Print and shaded views of the part. All mm, measured from the part's lowest x, y and z. Give positions to 0.01 mm unless a question says otherwise; leave off trailing zeros. Order: outer loops, then holes, each group sorted by start corner. A loop starts at its lowest first (then second) coordinate and runs counter-clockwise, first axis right, second up. Notation, with made-up numbers: (42.25, -22) - (85.25, -22) arc R31 cw to (85.25, 13) - close; hole circle Ø7 at (20.25, 40.5). An arc over 180 degrees is marked (long way). Answer in a Markdown table with one row per item.
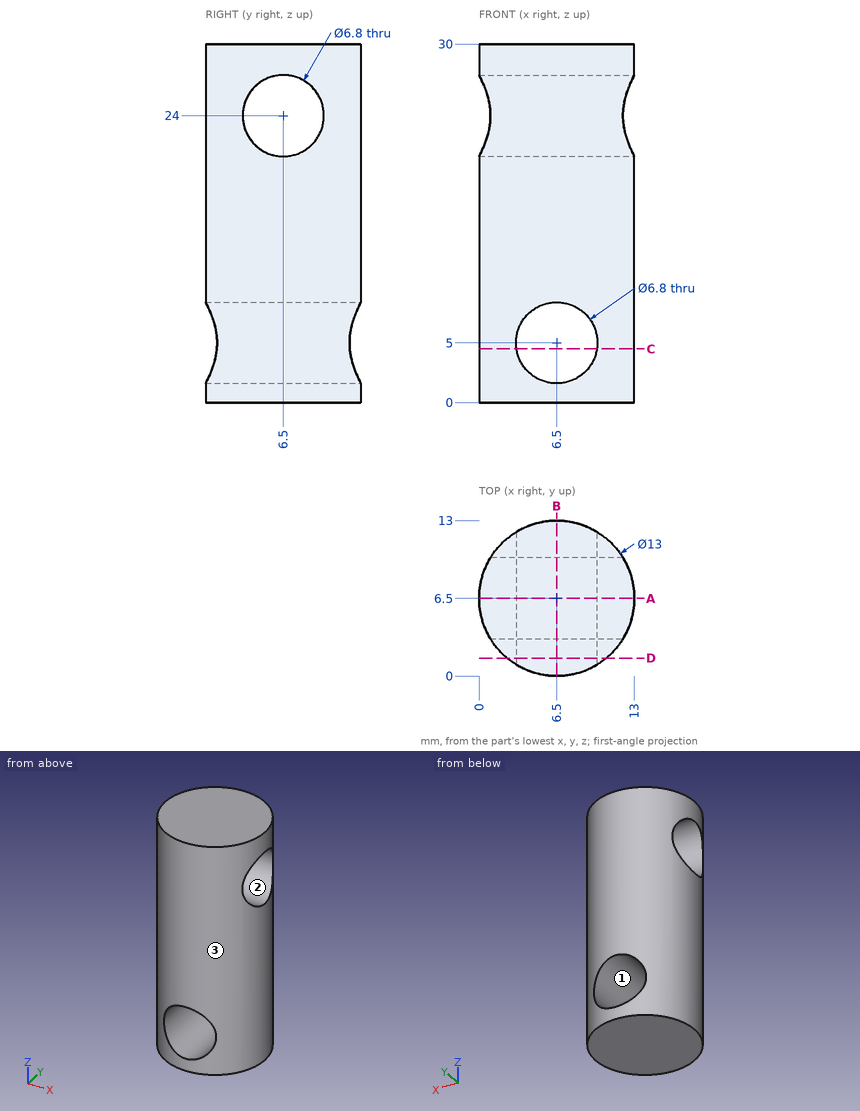
1. Two-plate mould, pull along X, no slides. Class the marked faces 1, 2 and 3: +X half, -X half, draft (parallel to the pull), parting line (faces both ways), or undercut.
Check result:
| item | result |
|---|---|
| face 1 | undercut |
| face 2 | draft |
| face 3 | parting line |
2. Drop flat-ended pins along their axis: P1, Ø4, axis at y = 2.5, z = 21, coming from the -X side; P2, Ø3, axis at y = 1.5, z = 5, coming from the +X side; P3, Ø4, axis at y = 7, z = 12.5, coming from the -X side; P4, Ø6, axis at x = 6.5, z = 5, coming from the +Y side. Give the stop position or say it passes through.
Check result:
| item | result |
|---|---|
| P1 | stops at x = 0.32 |
| P2 | stops at x = 11.98 |
| P3 | stops at x = 0 |
| P4 | passes through |
3. Cut at B-B on x = 6.5. Write the cut outline in (y, z), and give its area (3 significant figures).
Check result:
| item | result |
|---|---|
| outline | (0, 0) - (13, 0) - (13, 1.6) - (0, 1.6) - close; (0, 8.4) - (13, 8.4) - (13, 30) - (0, 30) - close; hole circle Ø6.8 at (6.5, 24) |
| area | 265 mm² |
4. Probe line 1 (Z direction, x = 6.5, y = 6.5); line 2 (Z direction, x = 6.5, y = 8.5); line 3 (Z direction, x = 10, y = 6.5). List the from-to ranges inside material, lowest first.
Check result:
| item | result |
|---|---|
| line 1 | z = 0 to 1.6, 8.4 to 20.6, 27.4 to 30 |
| line 2 | z = 0 to 1.6, 8.4 to 21.25, 26.75 to 30 |
| line 3 | z = 0 to 20.6, 27.4 to 30 |
5. Cut at D-D on y = 1.5. Write the cut outline in (x, z).
Check result:
| item | result |
|---|---|
| outline | (2.35, 0) - (10.65, 0) - (10.65, 30) - (2.35, 30) - close; hole circle Ø6.8 at (6.5, 5) |
6. Cut at C-C on z = 4.5. Write the cut outline in (x, y).
Check result:
| item | result |
|---|---|
| outline | (3.14, 0.94) - (3.14, 12.06) arc R6.5 ccw to start; (9.86, 0.94) arc R6.5 ccw to (9.86, 12.06) - close |
7. Cut at A-A on y = 6.5. Write the cut outline in (x, z).
Check result:
| item | result |
|---|---|
| outline | (0, 0) - (13, 0) - (13, 20.6) - (0, 20.6) - close; (0, 27.4) - (13, 27.4) - (13, 30) - (0, 30) - close; hole circle Ø6.8 at (6.5, 5) |
